Build history of the part. All positions in model axes, mm. A direction names the side the tool comes from. Round coordinates to 2 decimals unless told otherwise and drop trailing zeros. Order: outer loops, then holes, each group sorted by start corner. A loop starts at its lowest first (then second) coordinate and runs counter-clockwise, first axis right, second up. Notation, with made-up numbers: (11.25, 66.5) -> (52.25, 66.5) arc R18 ccw to (52.25, 70.5) -> close; hole circle Ø9 at (56.25, -38.5). An arc over 180 degrees is marked (long way). Write item = value, one per line.
from build123d import *

# Parameters (mm, degrees)
F0_W     = 50.8
F0_H     = 50.8
F0_R     = 11.629438
F1_DEPTH = 50.8
F2_W     = 18.713556
F2_H     = 20.050238
F3_DEPTH = 25.4
F4_R     = 11.069142
F5_DEPTH = 25.4


with BuildPart() as f1:
    # F0 (on Front) → F1 (new body)
    with BuildSketch(Plane.XZ):
        with Locations((25.4, 25.4)):
            Rectangle(F0_W, F0_H)
        with Locations((25.4, 25.4)):
            Circle(F0_R, mode=Mode.SUBTRACT)
    extrude(amount=F1_DEPTH)

    # F2 (on face) → F3 (join)
    with BuildSketch(Plane(origin=(0, 0, 0), x_dir=(1, 0, 0), z_dir=(0, 0, -1))):
        with Locations((27.306516, 27.974857)):
            Rectangle(F2_W, F2_H)
    extrude(amount=F3_DEPTH)

    # F4 (on face) → F5 (join)
    with BuildSketch(Plane.YZ.offset(50.8)):
        with Locations((-25.4, 25.4)):
            Circle(F4_R)
    extrude(amount=F5_DEPTH)


solid = f1.part
Q1. Probe probe 1 along Z at (x, y) = (25, -25); probe 2 along X at (y, z) = (-29.5, 3); probe 3 along Z at (x, y) = (25.4, -17). List the from-to ranges inside material, lowest first.
Check values:
probe_1 = -25.4 to 13.78, 37.02 to 50.8
probe_2 = 0 to 50.8
probe_3 = 0 to 13.77, 37.03 to 50.8
Q2. Cut at D-D, the plane x = 66. List the corners of the cut face in (y, z).
Check values:
outline = circle Ø22.14 at (-25.4, 25.4)
Q3. Cut at B-B, the plane x = 25.4. List the corners of the cut face in (y, z), and give its area (3 significant figures).
Check values:
outline = (-50.8, 0) -> (-38, 0) -> (-38, -25.4) -> (-17.95, -25.4) -> (-17.95, 0) -> (0, 0) -> (0, 13.77) -> (-50.8, 13.77) -> close; (-50.8, 37.03) -> (0, 37.03) -> (0, 50.8) -> (-50.8, 50.8) -> close
area = 1,910 mm²
Q4. Which spindle directions (+Z, -Z, +X, -X, +Y, -Y) get a long thin tool onto all of the face, cutting with end or side? Do faces 1 (the face through (50.8, -14, 25)), 2 (the face through (27, -38, -13)), 3 (the face through (17.95, -28, -13)). Say none if no direction does.
Check values:
face_1 = +X
face_2 = -Z, +X, -X, -Y
face_3 = -Z, -X, +Y, -Y
Q5. Cut at C-C, the plane y = -25.4. List the corners of the cut face in (x, z).
Check values:
outline = (0, 0) -> (17.95, 0) -> (17.95, -25.4) -> (36.66, -25.4) -> (36.66, 0) -> (50.8, 0) -> (50.8, 14.33) -> (76.2, 14.33) -> (76.2, 36.47) -> (50.8, 36.47) -> (50.8, 50.8) -> (0, 50.8) -> close; hole circle Ø23.26 at (25.4, 25.4)
Q6. Cut at A-A, the plane z = 25.4. List the corners of the cut face in (x, y), and give its area (3 significant figures).
Check values:
outline = (0, -50.8) -> (13.77, -50.8) -> (13.77, 0) -> (0, 0) -> close; (37.03, -50.8) -> (50.8, -50.8) -> (50.8, -36.47) -> (76.2, -36.47) -> (76.2, -14.33) -> (50.8, -14.33) -> (50.8, 0) -> (37.03, 0) -> close
area = 1,960 mm²
Q7. Flat gauge pins, fed straight in: pin 1 (3 mm diameter, centred on x = 39.5, y = -10.5, fed in from -Z); pin 2 (6 mm diameter, centred on x = 31, z = -8, fed in from +Y); pin 3 (3 mm diameter, centred on y = -6, z = -2.5, fed in from +X); pin 4 (16 mm diameter, centred on y = -23, z = -15, fed in from +X). Where does each tip first touch, or does it go through?
Check values:
pin_1 = 0
pin_2 = -17.95
pin_3 = through
pin_4 = 36.66
